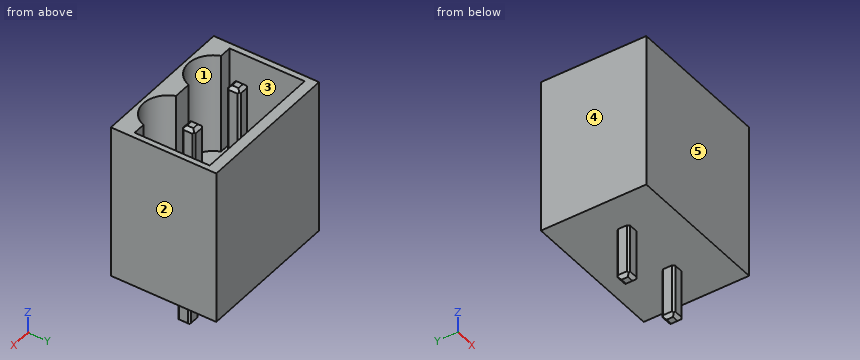
```python
from build123d import *

# Parameters (mm, degrees)
SKETCH_1_W          = 11.4
SKETCH_1_H          = 8.2
EXTRUDE_1_DEPTH     = 12.1
SKETCH_4_R          = 1.25
CUT_EXTRUDE_3_DEPTH = 8
CUT_EXTRUDE_4_DEPTH = 7.8
SKETCH_7_W          = 1
SKETCH_7_H          = 1
EXTRUDE_2_DEPTH     = 8
CHAMFER_1_SIZE      = 0.15
CHAMFER_2_SIZE      = 0.25
SKETCH_9_W          = 1
SKETCH_9_H          = 1
EXTRUDE_4_DEPTH     = 4
CHAMFER_5_SIZE      = 0.15
CHAMFER_6_SIZE      = 0.25


with BuildPart() as part:
    # Эскиз1 → Бобышка-Вытянуть1 (new body)
    with BuildSketch(Plane.XY):
        Rectangle(SKETCH_1_W, SKETCH_1_H)
    extrude(amount=EXTRUDE_1_DEPTH)

    # Эскиз4 → Вырез-Вытянуть3 (cut)
    with BuildSketch(Plane.XY.offset(12.1)):
        with Locations((-2.5, 0)):
            Circle(SKETCH_4_R)
        with Locations((2.5, 0)):
            Circle(SKETCH_4_R)
    extrude(amount=-CUT_EXTRUDE_3_DEPTH, mode=Mode.SUBTRACT)

    # Эскиз5 → Вырез-Вытянуть4 (cut)
    with BuildSketch(Plane.XY.offset(12.1)):
        with BuildLine():
            Line((-5.245621634, 0), (-5.245621634, 3.292901982))
            Line((-5.245621634, 3.292901982), (5.278509544, 3.292901982))
            Line((5.278509544, 3.292901982), (5.278509544, -2.548957219))
            Line((5.278509544, -2.548957219), (4.30582632, -2.548957219))
            ThreePointArc((4.30582632, -2.548957219), (2.5, -3.818893996), (0.69417368, -2.548957219))
            Line((0.69417368, -2.548957219), (-0.69417368, -2.548957219))
            ThreePointArc((-0.69417368, -2.548957219), (-2.5, -3.818893996), (-4.30582632, -2.548957219))
            Line((-4.30582632, -2.548957219), (-5.245621634, -2.548957219))
            Line((-5.245621634, -2.548957219), (-5.245621634, 0))
        make_face()
    extrude(amount=-CUT_EXTRUDE_4_DEPTH, mode=Mode.SUBTRACT)

    # Эскиз7 → Бобышка-Вытянуть2 (add)
    with BuildSketch(Plane.XY.offset(4.1)):
        with Locations((2.5, 0)):
            Rectangle(SKETCH_7_W, SKETCH_7_H)
        with Locations((-2.5, 0)):
            Rectangle(SKETCH_7_W, SKETCH_7_H)
    extrude(amount=EXTRUDE_2_DEPTH)

    # Фаска1
    chamfer_1_edges = [part.edges().sort_by_distance(p)[0] for p in [
        (-2, -0.5, 8.1),
        (-2, 0.5, 8.1),
        (-3, 0.5, 8.1),
        (-3, -0.5, 8.1),
        (3, -0.5, 8.1),
        (3, 0.5, 8.1),
        (2, 0.5, 8.1),
        (2, -0.5, 8.1),
    ]]
    chamfer(chamfer_1_edges, length=CHAMFER_1_SIZE)

    # Фаска2
    # the kernel refuses this chamfer: 0.25 mm, written as the material it takes off along each edge
    with BuildSketch(Plane(origin=(2, -0.992920747, 12.1), x_dir=(-0.027495876610586414, 0, -0.9996219169112968), z_dir=(0, 1, 0)), Plane(origin=(1.507079253, 0.5, 12.1), x_dir=(0, 0.027495876610586414, -0.9996219169112968), z_dir=(1, 0, 0)), Plane(origin=(3, 0.992920747, 12.1), x_dir=(0.02749587661058555, 0, -0.9996219169112968), z_dir=(0, -1, 0)), Plane(origin=(3.492920747, -0.5, 12.1), x_dir=(0, -0.027495876610586414, -0.9996219169112968), z_dir=(-1, 0, 0)), Plane(origin=(-2, 0.992920747, 12.1), x_dir=(0.027495876610586414, 0, -0.9996219169112968), z_dir=(0, -1, 0)), Plane(origin=(-1.507079253, -0.5, 12.1), x_dir=(0, -0.027495876610586414, -0.9996219169112968), z_dir=(-1, 0, 0)), Plane(origin=(-3, -0.992920747, 12.1), x_dir=(-0.02749587661058555, 0, -0.9996219169112968), z_dir=(0, 1, 0)), Plane(origin=(-3.492920747, 0.5, 12.1), x_dir=(0, 0.027495876610586414, -0.9996219169112968), z_dir=(1, 0, 0))) as chamfer_2_piece_1:
        Polygon((CHAMFER_2_SIZE * 0.999621916911, -CHAMFER_2_SIZE * 0.0274958766106), (-CHAMFER_2_SIZE * 0.0274958766106, -CHAMFER_2_SIZE * 0.999621916911), (0, 0), align=None)
    extrude(amount=1.985841494, mode=Mode.SUBTRACT)

    # Эскиз9 → Бобышка-Вытянуть4 (add)
    with BuildSketch(Plane(origin=(0, 0, 0), x_dir=(-1, 0, 0), z_dir=(0, 0, -1))):
        with Locations((2.5, -0.35)):
            Rectangle(SKETCH_9_W, SKETCH_9_H)
        with Locations((-2.5, -0.35)):
            Rectangle(SKETCH_9_W, SKETCH_9_H)
    extrude(amount=EXTRUDE_4_DEPTH)

    # Фаска5
    chamfer_5_edges = [part.edges().sort_by_distance(p)[0] for p in [
        (2, -0.85, -2),
        (2, 0.15, -2),
        (3, 0.15, -2),
        (3, -0.85, -2),
        (-3, -0.85, -2),
        (-3, 0.15, -2),
        (-2, 0.15, -2),
        (-2, -0.85, -2),
    ]]
    chamfer(chamfer_5_edges, length=CHAMFER_5_SIZE)

    # Фаска6
    # the kernel refuses this chamfer: 0.25 mm, written as the material it takes off along each edge
    with BuildSketch(Plane(origin=(-3.492920747, -0.85, -4), x_dir=(0, -0.02749587661058651, 0.9996219169112968), z_dir=(1, 0, 0)), Plane(origin=(1.507079253, -0.85, -4), x_dir=(0, -0.02749587661058651, 0.9996219169112968), z_dir=(1, 0, 0)), Plane(origin=(3, -1.342920747, -4), x_dir=(0.027495876610585647, 0, 0.9996219169112968), z_dir=(0, 1, 0)), Plane(origin=(2, 0.642920747, -4), x_dir=(-0.02749587661058651, 0, 0.9996219169112968), z_dir=(0, -1, 0)), Plane(origin=(-2, -1.342920747, -4), x_dir=(0.02749587661058651, 0, 0.9996219169112968), z_dir=(0, 1, 0)), Plane(origin=(-3, 0.642920747, -4), x_dir=(-0.027495876610585647, 0, 0.9996219169112968), z_dir=(0, -1, 0)), Plane(origin=(-1.507079253, 0.15, -4), x_dir=(0, 0.027495876610586403, 0.9996219169112968), z_dir=(-1, 0, 0)), Plane(origin=(3.492920747, 0.15, -4), x_dir=(0, 0.027495876610586403, 0.9996219169112968), z_dir=(-1, 0, 0))) as chamfer_6_piece_1:
        Polygon((CHAMFER_6_SIZE * 0.999621916911, -CHAMFER_6_SIZE * 0.0274958766106), (-CHAMFER_6_SIZE * 0.0274958766106, -CHAMFER_6_SIZE * 0.999621916911), (0, 0), align=None)
    extrude(amount=1.985841494, mode=Mode.SUBTRACT)


solid = part.part
```
Input: part model. Units: mm. Frame: model coordinates. Face numbers are marked on the shaded views. A direction names the side the tool comes from. Give positions to 0.01 mm unless a question says otherwise; leave off trailing zeros. Loops run counter-clockwise (first coordinate to the right, second up) from the corner with the lowest first, then second, coordinate; pieces in that order, holes last. Notation, with made-up numbers: M 19,-4 L 64,-4 A13 ccw 64,12 Z; hole C 63.25,27 d11. An arc over 180 degrees is marked long. Answer as CSV lines item,"result". Start each with the question number.
1. Pin query (flat end, axial travel): P1, Ø0.8, axis at y = -0.5, z = -1.5, coming from the -X side; P2, Ø0.8, axis at x = -2.5, z = -1.5, coming from the -Y side; P3, Ø0.8, axis at y = 0, z = -1, coming from the +X side. Return the tip coordinate at first contact, or that it passes through.
2. Line query: L1, parallel to Y at x = -2.5, z = 4.2; L2, parallel to X at y = -3.5, z = 7.75; L3, parallel to X at y = -1.5, z = 11.25. Output: solid intervals per line, ascending.
3. Section A-A on z = 8. Return loops of the section in (x, y), plus the area to 3 significant figures.
4. Section B-B on y = 1. Return loops of the section in (x, z).
5. Reachability of the marked faces 1 and 2 from +Z, -Z, +X, -X, +Y, -Y: full face, straight path, thin tool, end or side. Return the list, or none.
6. Section C-C on x = 2.5. Return loops of the section in (y, z).
7. Section D-D on y = 2.25. Return loops of the section in (x, z), plus the area to 3 significant figures.
8. Pull-direction query (X, two-part tool) for the marked faces 3, 4 and 5; classes: released by +X, released by -X, zero draft, split by the parting line, or undercut.
Computed values:
1,P1,"stops at x = -3"
1,P2,"stops at y = -0.85"
1,P3,"stops at x = 3"
2,L1,"y = -4.1 to -1.25, -0.5 to 0.5, 1.25 to 4.1"
2,L2,"x = -5.7 to -3.56, -1.44 to 1.44, 3.56 to 5.7"
2,L3,"x = -5.7 to -5.25, 5.28 to 5.7"
3,outline,"M -5.7,-4.1 L 5.7,-4.1 L 5.7,4.1 L -5.7,4.1 Z; M -3,-0.35 L -2.85,-0.5 L -2.15,-0.5 L -2,-0.35 L -2,0.35 L -2.15,0.5 L -2.85,0.5 L -3,0.35 Z; M 2,-0.35 L 2.15,-0.5 L 2.85,-0.5 L 3,-0.35 L 3,0.35 L 2.85,0.5 L 2.15,0.5 L 2,0.35 Z; hole M -5.25,-2.55 L -4.31,-2.55 A1.92 ccw -0.69,-2.55 L 0.69,-2.55 A1.92 ccw 4.31,-2.55 L 5.28,-2.55 L 5.28,3.29 L -5.25,3.29 Z"
3,area,"27.2 mm²"
4,outline,"M -5.7,0 L 5.7,0 L 5.7,12.1 L 5.28,12.1 L 5.28,4.3 L 3.25,4.3 L 3.25,4.1 L 1.75,4.1 L 1.75,4.3 L -1.75,4.3 L -1.75,4.1 L -3.25,4.1 L -3.25,4.3 L -5.25,4.3 L -5.25,12.1 L -5.7,12.1 Z"
5,face 1,"+Z"
5,face 2,"+Z, -Z, +X, +Y, -Y"
6,outline,"M -4.1,0 L -0.85,0 L -0.85,-3.75 L -0.6,-4 L -0.1,-4 L 0.15,-3.75 L 0.15,0 L 4.1,0 L 4.1,12.1 L 3.29,12.1 L 3.29,4.3 L 1.25,4.3 L 1.25,4.1 L 0.5,4.1 L 0.5,11.85 L 0.25,12.1 L -0.25,12.1 L -0.5,11.85 L -0.5,4.1 L -1.25,4.1 L -1.25,4.3 L -3.82,4.3 L -3.82,12.1 L -4.1,12.1 Z"
7,outline,"M -5.7,0 L 5.7,0 L 5.7,12.1 L 5.28,12.1 L 5.28,4.3 L -5.25,4.3 L -5.25,12.1 L -5.7,12.1 Z"
7,area,"55.9 mm²"
8,face 3,"undercut"
8,face 4,"released by -X"
8,face 5,"zero draft"
